```python
from build123d import *

# Parameters (mm, degrees)
BOSS_EXTRUDE1_DEPTH = 489
CUT_EXTRUDE2_DEPTH  = 485


with BuildPart() as part:
    # Sketch1 → Boss-Extrude1 (new body)
    with BuildSketch(Plane.XY):
        Polygon((0, 20), (0, 0), (20, 0), (20, 2), (2, 2), (2, 20), align=None)
    extrude(amount=BOSS_EXTRUDE1_DEPTH)

    # Sketch2 → Cut-Extrude2 (cut)
    with BuildSketch(Plane(origin=(0, 20, 0), x_dir=(1, 0, 0), z_dir=(0, 1, 0))):
        Polygon((2, 0), (0, 0), (2, -2), align=None)
        Polygon((2, 0), (2, -2), (20, -20), (20, 0), align=None)
        Polygon((2, -489), (2, -487), (0, -489), align=None)
        Polygon((20, -469), (2, -487), (2, -489), (20, -489), align=None)
    extrude(amount=-CUT_EXTRUDE2_DEPTH, mode=Mode.SUBTRACT)


solid = part.part
```
Work out the finished part from the listing and answer in its coordinate system (mm). A direction names the side the tool comes from. Coordinates: 2 decimals unless noted, no trailing zeros. Loops run counter-clockwise (first coordinate to the right, second up) from the corner with the lowest first, then second, coordinate; pieces in that order, holes last. Notation, with made-up numbers: (71, 31.5) - (79, 31.5) arc R17 cw to (79, 60.5) - close; hole circle Ø11 at (58.25, -9.75). An arc over 180 degrees is marked (long way). Use a Markdown table: item, result.
Item 1: Given pin 1 Ø12 at (x, z) = (12.5, 267.5) entering from +Y; pin 2 Ø12 at (x, z) = (8.5, 422.5) entering from -Y; pin 3 Ø1.5 at (y, z) = (4.5, 400.5) entering from +X, each flat-ended and moving along its own axis, determine where each tip first touches the part or whether it passes through.
Evaluation:
| item | result |
|---|---|
| pin 1 | stops at y = 2 |
| pin 2 | stops at y = 0 |
| pin 3 | stops at x = 2 |
Item 2: Find section A-A, the plane x = 6.5. Determine the outline of the cut face in (y, z), and give its area (3 significant figures).
Evaluation:
| item | result |
|---|---|
| outline | (0, 6.5) - (2, 6.5) - (2, 482.5) - (0, 482.5) - close |
| area | 952 mm2 |
Item 3: Find section C-C, the plane y = 11.5. Determine the outline of the cut face in (x, z).
Evaluation:
| item | result |
|---|---|
| outline | (0, 0) - (2, 2) - (2, 487) - (0, 489) - close |
Item 4: For faces 1 (the flat face through (6, 1, 6)), 2 (the flat face through (11, 2, 241)), determine the directions among +Z, -Z, +X, -X, +Y, -Y from which every point of the face is accessible in a straight line to the end or side of a thin tool.
Evaluation:
| item | result |
|---|---|
| face 1 | -Z, +X, +Y, -Y |
| face 2 | +Z, -Z, +X, +Y |
Item 5: Find section B-B, the plane z = 149. Determine the outline of the cut face in (x, y).
Evaluation:
| item | result |
|---|---|
| outline | (0, 0) - (20, 0) - (20, 2) - (2, 2) - (2, 20) - (0, 20) - close |
Item 6: Consider probe 1 along X at (y, z) = (6.5, 213.5); probe 2 along Z at (x, y) = (1.5, 15.75). Determine where each line is inside the solid, lowest interval first. Write a range as from..to.
Evaluation:
| item | result |
|---|---|
| probe 1 | x = 0..2 |
| probe 2 | z = 1.5..487.5 |
